Could you check a few things on this model? Use its own coordinates, in mm. A direction names the side the tool comes from. Coordinates: 2 decimals unless noted, no trailing zeros. Loops run counter-clockwise (first coordinate to the right, second up) from the corner with the lowest first, then second, coordinate; pieces in that order, holes last. Notation, with made-up numbers: (-39.5, -35) -> (12.5, -35) arc R13 ccw to (12.5, -11) -> close; hole circle Ø7 at (-9.75, 6). An arc over 180 degrees is marked (long way). One line per question, with ' | ' between items. Start each with the question number.
(1) Suppose I cut it at A-A (z = -3.75). Please give me the cut outline in (x, y), plus the area to 3 significant figures.
(2) Which directions (+Z, -Z, +X, -X, +Y, -Y) give clear straight access to the entire face, cutting with the end or side of a thin tool? Please do faces 4 (the face through (-2, 1.5, -2)), 5 (the face through (-0.88, 15.74, -1.99)), 6 (the face through (0, 7, -2)).
(3) Suppose I cut it at B-B (x = -3.45). Please give me the cut outline in (y, z).
(4) If we mould it in two halves opening along Z, with no side actions, what happens to faces 1 (the face through (-5, 7, -3)), 2 (the face through (-3, 7, 0)), 3 (the face through (-4.12, 0.74, -3.01))? For each: pulls with the +Z half, pulls with the -Z half, needs draft (parallel to the pull), parting line crosses it, or undercut.
(5) I'm going to push a flat-ended pin straight in: pin 1 Ø1.7 at (x, z) = (-3, -2) entering from -Y. Where does the tip first touch, or does it pass through?
(6) If I drill on line 1 along Z through (x, y) = (-2.5, 1.25); line 2 along Y through (x, z) = (-1.6, -1.45); line 3 along Y through (x, z) = (-3.65, -0.5), over which ranges is the centre line in solid material (lowest first)?
Autodesk Inventor part; units mm, degrees
ref_plane "YZ Plane" through (0, 0, 0) normal (1, 0, 0) x (0, 1, 0)
ref_plane "XZ Plane" through (0, 0, 0) normal (0, 1, 0) x (-1, 0, 0)
ref_plane "XY Plane" through (0, 0, 0) normal (0, 0, 1) x (1, 0, 0)
sketch "草圖1" plane through (0, 0, 0) normal (0, 1, 0) x (-1, 0, 0)
  line L0 (5, 0) -> (0, 0)
  line L1 (0, 0) -> (0, -5)
  line L2 (0, -5) -> (5, -5)
  line L3 (5, -5) -> (5, 0)
  circle A0 centre (2.5, -2.5) radius 1.7
  point P0 (2.5, -5)
  point P1 (5, -2.5)
  dimension "d0" = 5
  dimension "d1" = 5
  dimension "d2" = 3.4
extrude "擠出1" add sketch "草圖1" along normal blind 15 contours L3 L2 L1 L0 | A0
extrude "擠出2" cut sketch "草圖1" along normal blind 1.5 contours A0
sketch "草圖2" plane through (0, 15, 0) normal (0, 1, 0) x (1, 0, 0)
  circle A0 centre (-2.5, 2.5) radius 1.7
  point P0 (0, 0)
extrude "擠出3" add sketch "草圖2" along normal blind 1.5
sketch "草圖3" plane through (0, 0, 0) normal (1, 0, 0) x (0, 1, 0)
  line L0 (8.7779, 7.7621) -> (6.2221, 7.7621)
  line L1 (6.2221, 7.7621) -> (6.2221, -14.483)
  line L2 (6.2221, -14.483) -> (8.7779, -14.483)
  line L3 (8.7779, -14.483) -> (8.7779, 7.7621)
  line L4 (0, -5) -> (15, -5)
  point P0 (0, 0)
  point P1 (7.5, -14.483)
  point P2 (7.5, -5)
split_face "分割1"
properties part number "110033226_ipt_24_直條(3x1)"
Checks:
1) outline: (-5, 0) -> (-3.65, 0) -> (-3.65, 1.5) -> (-1.35, 1.5) -> (-1.35, 0) -> (0, 0) -> (0, 15) -> (-1.35, 15) -> (-1.35, 16.5) -> (-3.65, 16.5) -> (-3.65, 15) -> (-5, 15) -> close | area: 75.0 mm^2
2) face 4: -Y | face 5: +Y | face 6: +Z, -Z, +X, +Y, -Y
3) outline: (0, -5) -> (15, -5) -> (15, -3.91) -> (16.5, -3.91) -> (16.5, -1.09) -> (15, -1.09) -> (15, 0) -> (0, 0) -> (0, -1.09) -> (1.5, -1.09) -> (1.5, -3.91) -> (0, -3.91) -> close
4) face 1: needs draft | face 2: pulls with the +Z half | face 3: undercut
5) pin 1: stops at y = 1.5
6) line 1: z = -5 to -4.2, -0.8 to 0 | line 2: y = 1.5 to 16.5 | line 3: y = 0 to 15
